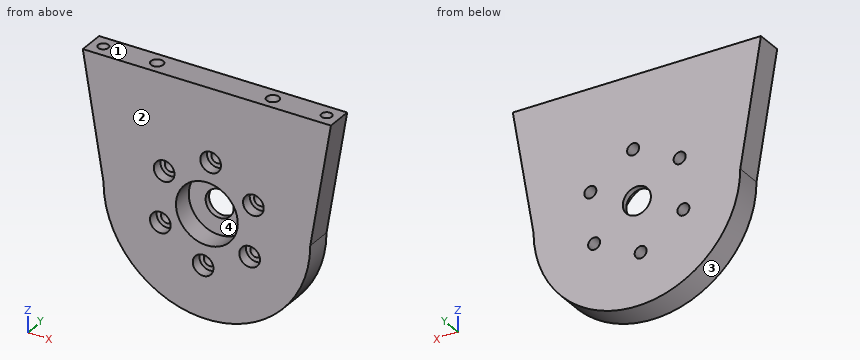
```python
from build123d import *

# Parameters (mm, degrees)
PLACA_J5_START           = -3.175
PLACA_J5_DEPTH           = 6.35
PLACA_J5_REDONDEO_START  = -3.175
CROQUIS9_R               = 25
PLACA_J5_REDONDEO_DEPTH  = 6.35
BARRENOS_SALIDA_M5_START = -3.175
CROQUIS10_R              = 1.45
CROQUIS10_R_2            = 3.4
BARRENOS_SALIDA_M5_DEPTH = 6.35
REFRENTADO_M2_5_START    = -3.175
CROQUIS11_R              = 2.5
REFRENTADO_M2_5_DEPTH    = 2.6
ROSCA_M3_CANTO_START     = 357.55
CROQUIS12_R              = 1.25
ROSCA_M3_CANTO_DEPTH     = 9
PASADORES_D3_START       = 359.55
CROQUIS13_R              = 1.5
PASADORES_D3_DEPTH       = 7
CROQUIS14_R              = 7.475
CORTAR_EXTRUIR1_DEPTH    = 5


with BuildPart() as part:
    # Croquis8 → Placa_J5 (new body)
    with BuildSketch(Plane(origin=(0, 0, 0), x_dir=(1, 0, 0), z_dir=(0, 1, 0)).offset(PLACA_J5_START)):
        Polygon((127.4, -336.55), (177.4, -336.55), (182.4, -366.55), (122.4, -366.55), align=None)
    extrude(amount=PLACA_J5_DEPTH)

    # Croquis9 → Placa_J5_redondeo (add)
    with BuildSketch(Plane(origin=(0, 0, 0), x_dir=(1, 0, 0), z_dir=(0, 1, 0)).offset(PLACA_J5_REDONDEO_START)):
        with Locations((152.4, -336.55)):
            Circle(CROQUIS9_R)
    extrude(amount=PLACA_J5_REDONDEO_DEPTH)

    # Croquis10 → Barrenos_salida_M5 (cut)
    with BuildSketch(Plane(origin=(0, 0, 0), x_dir=(1, 0, 0), z_dir=(0, 1, 0)).offset(BARRENOS_SALIDA_M5_START)):
        with Locations(Location((163.653984643, -341.990388742, 0), (0, 0, 270))):
            Circle(CROQUIS10_R)
        with Locations(Location((153.315477464, -349.016430965, 0), (0, 0, 270))):
            Circle(CROQUIS10_R)
        with Locations(Location((142.061492822, -343.576042223, 0), (0, 0, 270))):
            Circle(CROQUIS10_R)
        with Locations(Location((141.146015357, -331.109611258, 0), (0, 0, 270))):
            Circle(CROQUIS10_R)
        with Locations(Location((151.484522536, -324.083569035, 0), (0, 0, 270))):
            Circle(CROQUIS10_R)
        with Locations(Location((162.738507178, -329.523957777, 0), (0, 0, 270))):
            Circle(CROQUIS10_R)
        with Locations(Location((152.4, -336.55, 0), (0, 0, 270))):
            Circle(CROQUIS10_R_2)
    extrude(amount=BARRENOS_SALIDA_M5_DEPTH, mode=Mode.SUBTRACT)

    # Croquis11 → Refrentado_M2-5 (cut)
    with BuildSketch(Plane(origin=(0, 0, 0), x_dir=(1, 0, 0), z_dir=(0, 1, 0)).offset(REFRENTADO_M2_5_START)):
        with Locations(Location((163.653984643, -341.990388742, 0), (0, 0, 270))):
            Circle(CROQUIS11_R)
        with Locations(Location((153.315477464, -349.016430965, 0), (0, 0, 270))):
            Circle(CROQUIS11_R)
        with Locations(Location((142.061492822, -343.576042223, 0), (0, 0, 270))):
            Circle(CROQUIS11_R)
        with Locations(Location((141.146015357, -331.109611258, 0), (0, 0, 270))):
            Circle(CROQUIS11_R)
        with Locations(Location((151.484522536, -324.083569035, 0), (0, 0, 270))):
            Circle(CROQUIS11_R)
        with Locations(Location((162.738507178, -329.523957777, 0), (0, 0, 270))):
            Circle(CROQUIS11_R)
    extrude(amount=REFRENTADO_M2_5_DEPTH, mode=Mode.SUBTRACT)

    # Croquis12 → Rosca_M3_canto (cut)
    with BuildSketch(Plane.XY.offset(ROSCA_M3_CANTO_START)):
        with Locations((125.4, 0)):
            Circle(CROQUIS12_R)
        with Locations((179.4, 0)):
            Circle(CROQUIS12_R)
    extrude(amount=ROSCA_M3_CANTO_DEPTH, mode=Mode.SUBTRACT)

    # Croquis13 → Pasadores_D3 (cut)
    with BuildSketch(Plane.XY.offset(PASADORES_D3_START)):
        with Locations((138.4, 0)):
            Circle(CROQUIS13_R)
        with Locations((166.4, 0)):
            Circle(CROQUIS13_R)
    extrude(amount=PASADORES_D3_DEPTH, mode=Mode.SUBTRACT)

    # Croquis14 → Cortar-Extruir1 (cut)
    with BuildSketch(Plane.XZ.offset(3.175)):
        with Locations(Location((152.4, 336.55, 0), (0, 0, 270))):
            Circle(CROQUIS14_R)
    extrude(amount=-CORTAR_EXTRUIR1_DEPTH, mode=Mode.SUBTRACT)


solid = part.part
```
Build history of the part. All positions in model axes, mm. Face numbers are marked on the shaded views. Round coordinates to 2 decimals unless told otherwise and drop trailing zeros. Write each loop counter-clockwise with the first axis right and the second up, starting at its lowest first coordinate (ties: lowest second). Pieces come first, ordered by that corner, then holes. Notation, with made-up numbers: (8.25, 63.25) - (58.25, 63.25) arc R19 cw to (58.25, 98.25) - close; hole circle Ø10 at (31.5, 72). An arc over 180 degrees is marked (long way). Write each question's results on one line, items separated by ' | '. Start each with the question number.
Item 1: Drop flat-ended pins along their axis: P1, Ø4.5, axis at x = 163.65, z = 341.99, coming from the -Y side (3 decimals); P2, Ø1.5, axis at y = 2, z = 321.5, coming from the -X side; P3, Ø2, axis at y = 1.5, z = 342, coming from the -X side (3 decimals). Give the stop position or say it passes through.
Item 2: Saw through at C-C (z = 354.5). Write the cut outline in (x, y) (3 decimals), and give its area (3 significant figures).
Item 3: Mould opens along Z. For the marked faces 1, 2, 3 and 4 say: pulls with the +Z half, pulls with the -Z half, needs draft (parallel to the pull), parting line crosses it, or undercut.
Item 4: Saw through at A-A (z = 335). Write the cut outline in (x, y) (3 decimals), and give its area (3 significant figures).
Item 5: Wall check: L1, parallel to Y at x = 125.4, z = 361.5 (3 decimals); L2, parallel to X at y = 0.25, z = 331.5; L3, parallel to Z at x = 141, y = -1.5. Give the ranges that are in metal, low to high. Write a range as [from, to].
Item 6: Saw through at B-B (x = 125.4). Write the cut outline in (y, z) (3 decimals).
Results are:
1) P1: stops at y = -0.575 | P2: stops at x = 131.89 | P3: stops at x = 126.325
2) outline: (124.408, -3.175) - (180.392, -3.175) - (180.392, 3.175) - (124.408, 3.175) - close | area: 355 mm²
3) face 1: pulls with the +Z half | face 2: needs draft | face 3: pulls with the -Z half | face 4: undercut
4) outline: (127.448, -3.175) - (145.087, -3.175) - (145.087, 1.825) - (149.374, 1.825) - (149.374, 3.175) - (127.448, 3.175) - close; (155.426, 1.825) - (159.713, 1.825) - (159.713, -3.175) - (177.352, -3.175) - (177.352, 3.175) - (155.426, 3.175) - close | area: 236 mm²
5) L1: y = [-3.175, -1.25], [1.25, 3.175] | L2: x = [127.92, 139.75], [142.54, 146.89], [157.91, 176.88] | L3: z = [314.3, 328.61], [333.61, 341.31], [345.84, 366.55]
6) outline: (-3.175, 348.55) - (3.175, 348.55) - (3.175, 366.55) - (1.25, 366.55) - (1.25, 357.55) - (-1.25, 357.55) - (-1.25, 366.55) - (-3.175, 366.55) - close
